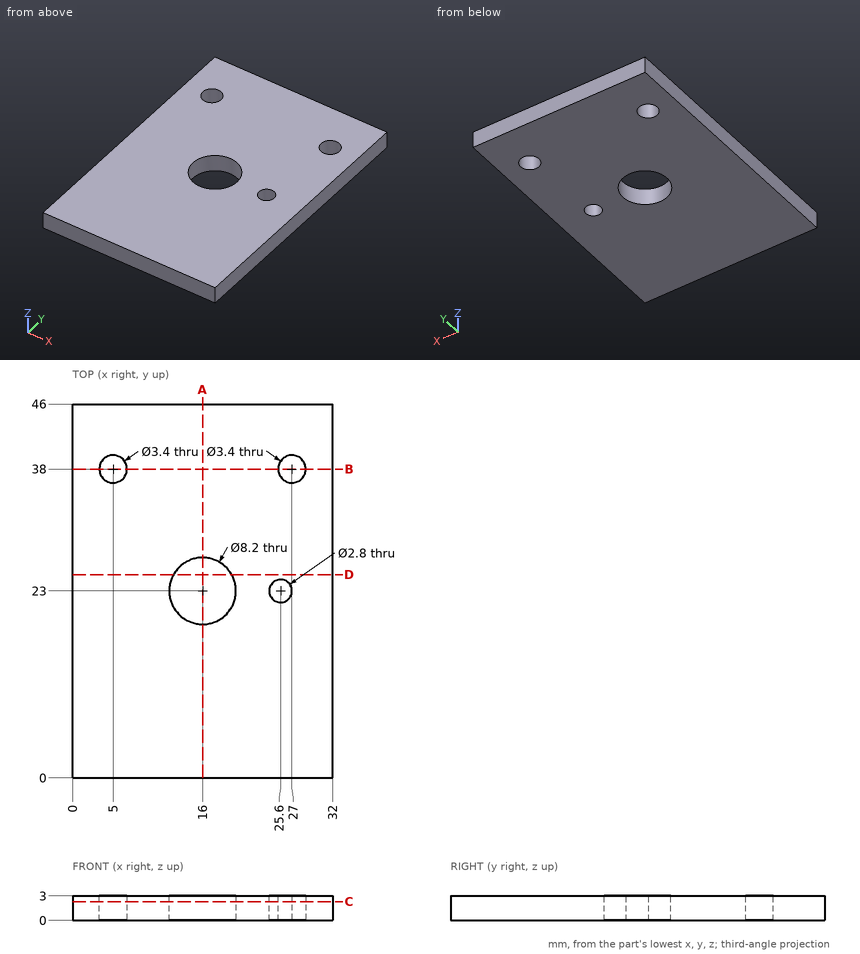
The figure shows three views and two pictorial views of one solid part (mm, origin at its lowest corner). Answer the questions. Coordinates: 2 decimals unless noted, no trailing zeros. Loops run counter-clockwise (first coordinate to the right, second up) from the corner with the lowest first, then second, coordinate; pieces in that order, holes last.
1) Find section B-B on y = 38. Write down the section's boundary in (x, z), then the cut area to 3 significant figures.
2) Find section A-A on x = 16. Write down the section's boundary in (y, z).
3) Find the intervals of material crossed by L1, parallel to Y at x = 26.5, z = 0.3; L2, parallel to Y at x = 25, z = 0.1; L3, parallel to Y at x = 25.6, z = 2.2, in increasing order.
4) Find section C-C on z = 2.3. Write down the section's boundary in (x, y), then the cut area to 3 significant figures.
5) Find section D-D on y = 25. Write down the section's boundary in (x, z), then the cut area to 3 significant figures.
Values:
1. outline: (0, 0) - (3.3, 0) - (3.3, 3) - (0, 3) - close; (6.7, 0) - (25.3, 0) - (25.3, 3) - (6.7, 3) - close; (28.7, 0) - (32, 0) - (32, 3) - (28.7, 3) - close
1. area: 75.6 mm2
2. outline: (0, 0) - (18.9, 0) - (18.9, 3) - (0, 3) - close; (27.1, 0) - (46, 0) - (46, 3) - (27.1, 3) - close
3. L1: y = 0 to 21.93, 24.07 to 36.38, 39.62 to 46
3. L2: y = 0 to 21.74, 24.26 to 46
3. L3: y = 0 to 21.6, 24.4 to 37.04, 38.96 to 46
4. outline: (0, 0) - (32, 0) - (32, 46) - (0, 46) - close; hole circle Ø3.4 at (5, 38); hole circle Ø8.2 at (16, 23); hole circle Ø2.8 at (25.6, 23); hole circle Ø3.4 at (27, 38)
4. area: 1,390 mm2
5. outline: (0, 0) - (12.42, 0) - (12.42, 3) - (0, 3) - close; (19.58, 0) - (32, 0) - (32, 3) - (19.58, 3) - close
5. area: 74.5 mm2
